Input: part model. Units: mm. Frame: model coordinates. A direction names the side the tool comes from. Round coordinates to 2 decimals unless told otherwise and drop trailing zeros. Loops run counter-clockwise (first coordinate to the right, second up) from the corner with the lowest first, then second, coordinate; pieces in that order, holes last.
1) Draft query along Z for faces 4 (the face through (3.986, -9.849, 17.725)), 5 (the face through (8, -26.289, -19)). Return one class per face: pulls with the +Z half, pulls with the -Z half, needs draft (parallel to the pull), parting line crosses it, or undercut.
2) Ray query, line 1 along Z through (x, y) = (3, -19.25); line 2 along Z through (x, y) = (9, -19.25); line 3 along X through (y, z) = (-21, -12.5). Return the intervals inside material, ascending.
3) First-contact query: pin 1 (2 mm diameter, centred on y = -13.5, z = -15, fed in from -X); pin 2 (2 mm diameter, centred on y = -9, z = -18.5, fed in from +X); pin 3 (3 mm diameter, centred on x = 9.5, y = -17, fed in from +Z). Flat tips, straight axial feed; report the tip coordinate or a pass-through.
4) Section B-B, the plane y = -15.5. Return loops of the section in (x, z).
5) Section C-C, the plane z = -13.5. Return loops of the section in (x, y).
6) Section A-A, the plane z = 0. Return loops of the section in (x, y).
7) Access query for faces 1 (the face through (-4, -10.287, -17)), 2 (the face through (-3.79, -9.41, -16.86)), 3 (the face through (6, -8.509, 17)). Directions: +Z, -Z, +X, -X, +Y, -Y. A direction counts if a zero-diameter tool reaches every point of the face in a straight line with its end or side. Return the directions, or none.
Autodesk Inventor part; units mm, degrees
ref_plane "Work Plane1" through (0, -8.509, -25.534) normal (-1, 0, 0) x (0, -1, 0)
ref_plane "YZ Plane" through (0, 0, 0) normal (1, 0, 0) x (0, 1, 0)
ref_plane "XZ Plane" through (0, 0, 0) normal (0, 1, 0) x (-1, 0, 0)
sketch "Sketch1" plane through (0, 0, 0) normal (1, 0, 0) x (0, 1, 0)
  line L0 (-8.509, -17.279) -> (-10.287, -17.279)
  line L1 (-10.287, -17.279) -> (-10.287, -18.168)
  line L2 (-10.287, -18.168) -> (-9.398, -18.168)
  line L3 (-9.398, -18.168) -> (-9.398, -20.454)
  line L4 (-9.398, -20.454) -> (-8.509, -20.454)
  line L5 (-8.509, 20.454) -> (-8.509, 17.279)
  line L6 (-8.509, 17.279) -> (-10.287, 17.279)
  line L7 (-10.287, 17.279) -> (-10.287, 18.168)
  line L8 (-10.287, 18.168) -> (-9.398, 18.168)
  line L9 (-9.398, 18.168) -> (-9.398, 20.454)
  line L10 (-8.509, 20.454) -> (-8.509, 25.534)
  line L11 (-8.509, 25.534) -> (-26.289, 25.534)
  line L12 (-26.289, 25.534) -> (-26.289, 20.454)
  line L13 (-26.289, 20.454) -> (-9.398, 20.454)
  line L14 (-8.509, -20.454) -> (-8.509, -25.534)
  line L15 (-8.509, -25.534) -> (-26.289, -25.534)
  line L16 (-26.289, -25.534) -> (-26.289, -20.454)
  line L17 (-26.289, -20.454) -> (-9.398, -20.454)
  line L18 (-26.289, 20.454) -> (-23.749, 20.454)
  line L19 (-8.509, -17.279) -> (-8.509, -20.454)
  line L20 (-8.509, -17.279) -> (-8.509, 17.279)
  line L21 (-8.509, 0) -> (-26.289, 0)
  dimension "d8" = 1.778
  dimension "d10" = 0.889
  dimension "d13" = 0.889
  dimension "d15" = 17.78
  dimension "d16" = 5.08
  dimension "d17" = 17.78
  dimension "d18" = 2.54
sketch "Sketch1 outline for Revolution1" plane through (0, 0, 0) normal (1, 0, 0) x (0, 1, 0)
  line L0 (-9.398, -18.168) -> (-9.398, -20.454)
  line L1 (-9.398, -20.454) -> (-26.289, -20.454)
  line L2 (-26.289, -20.454) -> (-26.289, -25.534)
  line L3 (-26.289, -25.534) -> (-8.509, -25.534)
  line L4 (-8.509, -25.534) -> (-8.509, -17.279)
  line L5 (-8.509, -17.279) -> (-10.287, -17.279)
  line L6 (-10.287, -17.279) -> (-10.287, -18.168)
  line L7 (-10.287, -18.168) -> (-9.398, -18.168)
  line L8 (-10.287, 17.279) -> (-8.509, 17.279)
  line L9 (-8.509, 17.279) -> (-8.509, 25.534)
  line L10 (-8.509, 25.534) -> (-26.289, 25.534)
  line L11 (-26.289, 25.534) -> (-26.289, 20.454)
  line L12 (-26.289, 20.454) -> (-9.398, 20.454)
  line L13 (-9.398, 20.454) -> (-9.398, 18.168)
  line L14 (-9.398, 18.168) -> (-10.287, 18.168)
  line L15 (-10.287, 18.168) -> (-10.287, 17.279)
revolve "Revolution1" add sketch "Sketch1 outline for Revolution1" angle 25 about axis through (0, -8.509, 0) along (0, 1, 0)
ref_plane "Work Plane1" through (0, -8.509, -25.534) normal (-1, 0, 0) x (0, -1, 0)
sketch "Sketch2" plane through (0, -8.509, -25.534) normal (-1, 0, 0) x (0, -1, 0)
  line L0 (0.889, 5.08) -> (17.78, 5.08)
  line L1 (17.78, 5.08) -> (17.78, 0)
  line L2 (0, 51.068) -> (17.78, 51.068)
  line L3 (17.78, 51.068) -> (0, 51.068)
  line L4 (-8.509, 25.534) -> (17.78, 25.534)
  line L5 (17.78, 51.068) -> (0, 51.068)
  line L6 (0, 51.068) -> (0, 45.988)
  line L7 (0, 45.988) -> (17.78, 45.988)
  line L8 (17.78, 45.988) -> (17.78, 51.068)
  line L9 (0.889, 5.08) -> (0, 5.08)
  line L10 (17.78, 5.08) -> (17.78, 0)
  line L11 (17.78, 2.392337) -> (17.78, 0)
  line L12 (17.78, 0) -> (0, 0)
  line L13 (0, 0) -> (0, 5.08)
  point P0 (0.889, 7.366)
sketch "Sketch2 outline for Revolution2" plane through (0, -8.509, -25.534) normal (-1, 0, 0) x (0, -1, 0)
  line L0 (17.78, 5.08) -> (0, 5.08)
  line L1 (0, 5.08) -> (0, 0)
  line L2 (0, 0) -> (17.78, 0)
  line L3 (17.78, 0) -> (17.78, 5.08)
  line L4 (17.78, 45.988) -> (17.78, 51.068)
  line L5 (0, 45.988) -> (17.78, 45.988)
  line L6 (0, 51.068) -> (0, 45.988)
  line L7 (17.78, 51.068) -> (0, 51.068)
revolve "Revolution2" add sketch "Sketch2 outline for Revolution2" angle 155 about axis through (0, 0, 0) along (0, -1, 0)
properties part number "RSL light mount (guard 1)"
Final values:
1. face 4: undercut
1. face 5: needs draft
2. line 1: z = -25.36 to -20.23, 20.23 to 25.36
2. line 2: z = -23.9 to -18.37, 18.37 to 23.9
2. line 3: x = -22.27 to -16.19, 16.19 to 22.27
3. pin 1: stops at x = -21.35
3. pin 2: stops at x = 18.59
3. pin 3: stops at z = 24.25
4. outline: circle Ø51.07 at (0, 0); hole circle Ø40.91 at (0, 0)
5. outline: (-21.67, -26.29) - (-15.37, -26.29) - (-15.37, -8.51) - (-21.67, -8.51) - close; (15.37, -26.29) - (21.67, -26.29) - (21.67, -8.51) - (15.37, -8.51) - close
6. outline: (-25.53, -26.29) - (-20.45, -26.29) - (-20.45, -8.51) - (-25.53, -8.51) - close; (20.45, -26.29) - (25.53, -26.29) - (25.53, -8.51) - (20.45, -8.51) - close
7. face 1: -Y
7. face 2: +Y, -Y
7. face 3: +Z, -Z, +X, -X, +Y
